Model file for the job. Use its own axes, mm. Round coordinates to 2 decimals unless told otherwise and drop trailing zeros. Loops run counter-clockwise (first coordinate to the right, second up) from the corner with the lowest first, then second, coordinate; pieces in that order, holes last. Notation, with made-up numbers: (80, 28.5) - (87, 28.5) arc R28 ccw to (87, 54.5) - close; hole circle Ø10 at (19.25, 42). An arc over 180 degrees is marked (long way). Answer as a JSON object with one key per item and string values.
from build123d import *

# Parameters (mm, degrees)
BOSS_EXTRUDE1_DEPTH = 2
SKETCH2_R           = 1.6
CUT_EXTRUDE1_DEPTH  = 10
SKETCH3_R           = 2
BOSS_EXTRUDE2_DEPTH = 15


with BuildPart() as part:
    # Sketch1 → Boss-Extrude1 (new body)
    with BuildSketch(Plane.XY):
        with BuildLine():
            ThreePointArc((0, 10), (-10, 0), (0, -10))
            Line((0, -10), (60, -6))
            ThreePointArc((60, -6), (66, 0), (60, 6))
            Line((60, 6), (0, 10))
        make_face()
    extrude(amount=BOSS_EXTRUDE1_DEPTH)

    # Sketch2 → Cut-Extrude1 (cut)
    with BuildSketch(Plane.XY.offset(2)):
        with Locations((-4.977412632, 4.921926807)):
            Circle(SKETCH2_R)
        with Locations((4.921926807, 4.977412632)):
            Circle(SKETCH2_R)
        with Locations((4.977412632, -4.921926807)):
            Circle(SKETCH2_R)
        with Locations((-4.921926807, -4.977412632)):
            Circle(SKETCH2_R)
    extrude(amount=-CUT_EXTRUDE1_DEPTH, mode=Mode.SUBTRACT)

    # Sketch3 → Boss-Extrude2 (add)
    with BuildSketch(Plane.XY.offset(2)):
        with Locations((60, 0)):
            Circle(SKETCH3_R)
    extrude(amount=BOSS_EXTRUDE2_DEPTH)


solid = part.part
1) Slice it at C-C on y = 4.25. List the corners of the cut face in (x, z), then the cut area to 3 significant figures.
Values follow:
{"outline": "(-9.05, 0) - (-6.43, 0) - (-6.43, 2) - (-9.05, 2) - close; (-3.53, 0) - (3.5, 0) - (3.5, 2) - (-3.53, 2) - close; (6.35, 0) - (64.24, 0) - (64.24, 2) - (6.35, 2) - close", "area": "135 mm²"}
2) Slice it at A-A on y = 0. List the corners of the cut face in (x, z).
Values follow:
{"outline": "(-10, 0) - (66, 0) - (66, 2) - (62, 2) - (62, 17) - (58, 17) - (58, 2) - (-10, 2) - close"}
3) Drop flat-ended pins along their axis: P1, Ø4, axis at x = 24.5, y = 5.5, coming from the -Z side; P2, Ø3, axis at y = -4.5, z = 13, coming from the +X side; P3, Ø10, axis at x = 43, z = 6.5, coming from the -Y side; P4, Ø10, axis at x = 16, y = -2, coming from the +Z side. Give the stop position or say it passes through.
Values follow:
{"P1": "z = 0", "P2": "through", "P3": "y = -7.28", "P4": "z = 2"}
4) Slice it at B-B on z = 1. List the corners of the cut face in (x, y), then the cut area to 3 significant figures.
Values follow:
{"outline": "(0, -10) - (60, -6) arc R6 ccw to (60, 6) - (0, 10) arc R10 ccw to start; hole circle Ø3.2 at (-4.98, 4.92); hole circle Ø3.2 at (-4.92, -4.98); hole circle Ø3.2 at (4.92, 4.98); hole circle Ø3.2 at (4.98, -4.92)", "area": "1,140 mm²"}
5) Slice it at D-D on x = 57. List the corners of the cut face in (y, z), then the cut area to 3 significant figures.
Values follow:
{"outline": "(-6.2, 0) - (6.2, 0) - (6.2, 2) - (-6.2, 2) - close", "area": "24.8 mm²"}
6) Two-plate mould, pull along X, no slides. Class faces 1 (the flat face through (27, 0, 0)), 2 (the cylindrical face through (-5.186, 6.508, 1.014)), 3 (the cylindrical face through (58, 0, 9)): pulls with the +X half, pulls with the -X half, needs draft (parallel to the pull), parting line crosses it, or undercut.
Values follow:
{"face 1": "needs draft", "face 2": "undercut", "face 3": "parting line crosses it"}
7) Probe probe 1 along Y at (x, z) = (-5.5, 1.75); probe 2 along Z at (x, y) = (16, 2); probe 3 along X at (y, z) = (0.75, 15.5). List the from-to ranges inside material, lowest first.
Values follow:
{"probe 1": "-8.35 to -6.47, -3.49 to 3.41, 6.43 to 8.35", "probe 2": "0 to 2", "probe 3": "58.15 to 61.85"}
